```python
from build123d import *

# Parameters (mm, degrees)
F0_R            = 85
F1_DEPTH        = 2
F3_DEPTH        = 2
F3_COPIES_COUNT = 4
F4_R            = 2.95
F5_DEPTH        = 25


# Not quite as in the source:
# - a pattern or mirror of a feature is missing from the dataset's text; its kind, count and spacing are read off the source's solid
# - a feature names something its author has since deleted; it is built from what else it names


with BuildPart() as f1:
    # F0 (on Top) → F1 (new body)
    with BuildSketch(Plane.XY):
        Circle(F0_R)
    extrude(amount=F1_DEPTH)

    # F2 (on face) → F3 (join)
    with BuildSketch(Plane.XY.offset(2)):
        with BuildLine():
            ThreePointArc((-42.5, -73.6121593217), (-60.1040764009, -60.1040764009), (-73.6121593217, -42.5))
            Line((-73.6121593217, -42.5), (-86.6025403784, -50))
            ThreePointArc((-86.6025403784, -50), (-70.7106781187, -70.7106781187), (-50, -86.6025403784))
            Line((-50, -86.6025403784), (-42.5, -73.6121593217))
        make_face()
    f3 = extrude(amount=-F3_DEPTH)

    # F3_copies: F3 ×4 about axis
    f3_copies_axis = Axis((0, 0, 0), (0, 0, 1))
    for i in range(1, F3_COPIES_COUNT):
        add(f3.rotate(f3_copies_axis, i * 360 / F3_COPIES_COUNT))

    # F4 (on face) → F5 (cut)
    with BuildSketch(Plane(origin=(0, 0, 0), x_dir=(1, 0, 0), z_dir=(0, 0, -1))):
        Circle(F4_R)
    extrude(amount=-F5_DEPTH, mode=Mode.SUBTRACT)


solid = f1.part
```
Input: part model. Units: mm. Frame: model coordinates. A direction names the side the tool comes from. Give positions to 0.01 mm unless a question says otherwise; leave off trailing zeros. Loops run counter-clockwise (first coordinate to the right, second up) from the corner with the lowest first, then second, coordinate; pieces in that order, holes last. Notation, with made-up numbers: (2.25, 3.5) -> (13.25, 3.5) arc R32 cw to (13.25, 39.5) -> close; hole circle Ø3 at (17.5, -4.75). An arc over 180 degrees is marked (long way). Use a Markdown table: item, result.
Q1. First-contact query: P1, Ø4.5, axis at x = 0, y = 0, coming from the +Z side (1 decimal); P2, Ø1, axis at x = -13, z = 1, coming from the -Y side. Flat tips, straight axial feed; report the tip coordinate or a pass-through.
Entries:
| item | result |
|---|---|
| P1 | passes through |
| P2 | stops at y = -84.08 |
Q2. Section query C-C, the plane z = 1.7. Return the cut outline in (x, y), plus the area to 3 significant figures.
Entries:
| item | result |
|---|---|
| outline | (-86.6, -50) arc R100 ccw to (-50, -86.6) -> (-42.5, -73.61) arc R85 ccw to (42.5, -73.61) -> (50, -86.6) arc R100 ccw to (86.6, -50) -> (73.61, -42.5) arc R85 ccw to (73.61, 42.5) -> (86.6, 50) arc R100 ccw to (50, 86.6) -> (42.5, 73.61) arc R85 ccw to (-42.5, 73.61) -> (-50, 86.6) arc R100 ccw to (-86.6, 50) -> (-73.61, 42.5) arc R85 ccw to (-73.61, -42.5) -> close; hole circle Ø5.9 at (0, 0) |
| area | 25,600 mm² |
Q3. Section query D-D, the plane y = -53. Return the cut outline in (x, z), plus the area to 3 significant figures.
Entries:
| item | result |
|---|---|
| outline | (-84.8, 0) -> (84.8, 0) -> (84.8, 2) -> (-84.8, 2) -> close |
| area | 339 mm² |
Q4. Pull-direction query (X, two-part tool) for faces 6 (the flat face through (-46.302, -80.198, 1.014)), 7 (the flat face through (80.02, 46.2, 1.01)), 8 (the flat face through (-80.198, 46.303, 1.014)); classes: pulls with the +X half, pulls with the -X half, needs draft (parallel to the pull), parting line crosses it, or undercut.
Entries:
| item | result |
|---|---|
| face 6 | undercut |
| face 7 | pulls with the +X half |
| face 8 | pulls with the -X half |
Q5. Access query for faces 1 (the flat face through (-80.02, -46.2, 1.01)), 2 (the flat face through (46.2, -80.02, 1.01)), 3 (the flat face through (80.198, -46.303, 1.014)), 4 (the flat face through (46.303, 80.198, 1.014)), 5 (the cylindrical face through (70.45, -70.97, 1.01)). Directions: +Z, -Z, +X, -X, +Y, -Y. A direction counts if a zero-diameter tool reaches every point of the face in a straight line with its end or side. Return the directions, or none.
Entries:
| item | result |
|---|---|
| face 1 | +Z, -Z, -X |
| face 2 | +Z, -Z, -Y |
| face 3 | +Z, -Z, +X |
| face 4 | +Z, -Z, +Y |
| face 5 | +Z, -Z, +X, -Y |
Q6. Ray query, probe 1 along Y at (x, z) = (0, 0.7); probe 2 along X at (y, z) = (1.5, 0.2). Return the intervals inside material, ascending. Write a range as from..to.
Entries:
| item | result |
|---|---|
| probe 1 | y = -85..-2.95, 2.95..85 |
| probe 2 | x = -84.99..-2.54, 2.54..84.99 |
Q7. Section query A-A, the plane y = 0. Return the cut outline in (x, z), plus the area to 3 significant figures.
Entries:
| item | result |
|---|---|
| outline | (-85, 0) -> (-2.95, 0) -> (-2.95, 2) -> (-85, 2) -> close; (2.95, 0) -> (85, 0) -> (85, 2) -> (2.95, 2) -> close |
| area | 328 mm² |
